Part model, mm, in its own coordinate system. Face numbers are marked on the shaded views. A direction names the side the tool comes from. Coordinates: 2 decimals unless noted, no trailing zeros. Loops run counter-clockwise (first coordinate to the right, second up) from the corner with the lowest first, then second, coordinate; pieces in that order, holes last. Notation, with made-up numbers: M 84,80.5 L 140,80.5 A35 ccw 140,115.5 Z; hole C 74.5,68 d10. An arc over 180 degrees is marked long. Use a Markdown table: item, result. Add a question column.
1) Tool access for the marked faces 1 and 2: list every direction of +Z, -Z, +X, -X, +Y, -Y with a clear straight run to the whole face (end or side of a thin tool).
2) Band-saw the part on A-A (x = 0). List the corners of the cut face in (y, z), plus the area to 3 significant figures.
3) Wall check: probe 1 along X at (y, z) = (0, 15.25); probe 2 along Z at (x, y) = (6, -2.5); probe 3 along Y at (x, z) = (0, 14.25). Give the ranges that are in metal, low to high. Write a range as from..to.
4) Pull direction X, two halves, no side cores. Call the marked faces 3, 4 and 5: released by +X, released by -X, zero draft, split by the parting line, or undercut.
5) Band-saw the part on C-C (z = 3.25). List the corners of the cut face in (x, y), plus the area to 3 significant figures.
6) Band-saw the part on D-D (z = 20.5). List the corners of the cut face in (x, y), plus the area to 3 significant figures.
7) Pin check, flat tips, straight feed: pin 1 Ø1 at (y, z) = (-19, 5) entering from +X; pin 2 Ø8 at (y, z) = (-16, 20) entering from +X; pin 3 Ø10 at (y, z) = (9, 15) entering from -X. Stop position of each tip, or through.
8) Band-saw the part on B-B (y = 0). List the corners of the cut face in (x, z), plus the area to 3 significant figures.
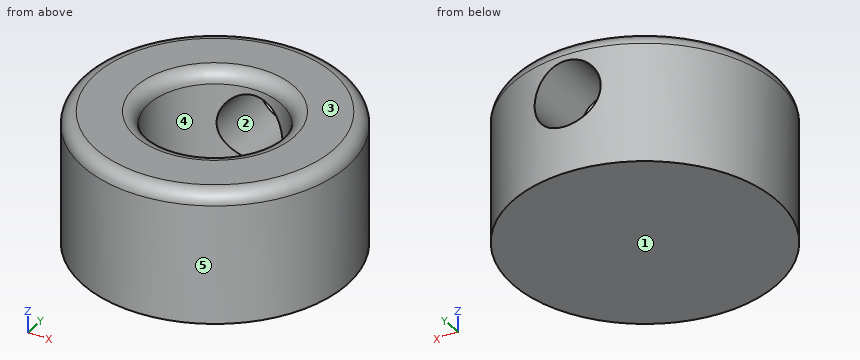
from build123d import *

# Parameters (mm, degrees)
F2_R     = 2.54
F3_R     = 6.35
F4_DEPTH = 25.401


with BuildPart() as f1:
    # F0 (on Front) → F1 (revolve)
    with BuildSketch(Plane.XZ):
        Polygon((0, 7.62), (0, 0), (25.4, 0), (25.4, 25.4), (12.7, 25.4), (12.7, 7.62), align=None)
    revolve(axis=Axis((0, 0, 3.81), (0, 0, -1)))

    # F2
    f2_edges = [f1.edges().sort_by_distance(p)[0] for p in [
        (-25.4, 0, 25.4),
        (-12.7, 0, 25.4),
    ]]
    fillet(f2_edges, radius=F2_R)

    # F3 (on Front) → F4 (cut, through all)
    with BuildSketch(Plane.XZ):
        with Locations((0, 15.365091)):
            Circle(F3_R)
    extrude(amount=-F4_DEPTH, mode=Mode.SUBTRACT)


solid = f1.part
Entries:
| question | item | result |
|---|---|---|
| 1 | face 1 | -Z, +X, -X, +Y, -Y |
| 1 | face 2 | +Y |
| 2 | outline | M -25.4,0 L 25.4,0 L 25.4,9.02 L 12.7,9.02 L 12.7,7.62 L -12.7,7.62 L -12.7,22.86 A2.54 ccw -15.24,25.4 L -22.86,25.4 A2.54 ccw -25.4,22.86 Z; M 12.7,21.72 L 25.4,21.72 L 25.4,22.86 A2.54 ccw 22.86,25.4 L 15.24,25.4 A2.54 ccw 12.7,22.86 Z |
| 2 | area | 672 mm2 |
| 3 | probe 1 | -25.4..-12.7, 12.7..25.4 |
| 3 | probe 2 | 0..7.62 |
| 3 | probe 3 | -25.4..-12.7 |
| 4 | face 3 | zero draft |
| 4 | face 4 | undercut |
| 4 | face 5 | split by the parting line |
| 5 | outline | C 0,0 d50.8 |
| 5 | area | 2,030 mm2 |
| 6 | outline | M -3.74,12.14 L -3.74,25.12 A25.4 ccw long 3.74,25.12 L 3.74,12.14 A12.7 cw long Z |
| 6 | area | 1,420 mm2 |
| 7 | pin 1 | x = 17.4 |
| 7 | pin 2 | x = 22.39 |
| 7 | pin 3 | x = -25.08 |
| 8 | outline | M -25.4,0 L 25.4,0 L 25.4,22.86 A2.54 ccw 22.86,25.4 L 15.24,25.4 A2.54 ccw 12.7,22.86 L 12.7,7.62 L -12.7,7.62 L -12.7,22.86 A2.54 ccw -15.24,25.4 L -22.86,25.4 A2.54 ccw -25.4,22.86 Z |
| 8 | area | 833 mm2 |
